For this review, take the finished solid that the model builds, in its own axes (mm). Face numbers are marked on the shaded views. A direction names the side the tool comes from. Give positions to 0.01 mm unless a question says otherwise; leave off trailing zeros. Loops run counter-clockwise (first coordinate to the right, second up) from the corner with the lowest first, then second, coordinate; pieces in that order, holes last. Notation, with made-up numbers: (46, -12.75) -> (88, -12.75) arc R21 ccw to (88, 3.25) -> close; hole circle Ø5 at (-25, 14). An arc over 180 degrees is marked (long way). Write each question's results on one line, items separated by ' | '. Start each with the question number.
```python
from build123d import *

# Parameters (mm, degrees)
SKETCH1_R           = 1.7
BOSS_EXTRUDE1_DEPTH = 34.5
CUT_EXTRUDE1_DEPTH  = 20.5
CUT_EXTRUDE2_START  = -7
CUT_EXTRUDE2_DEPTH  = 7


with BuildPart() as part:
    # Sketch1 → Boss-Extrude1 (new body)
    with BuildSketch(Plane.XY):
        with BuildLine():
            Line((-1.71, 8.48), (5.42, 8.48))
            ThreePointArc((5.42, 8.48), (8.934320702, 7.024320703), (10.39, 3.51))
            Line((10.39, 3.51), (10.39, -3.510005593))
            ThreePointArc((10.39, -3.510005593), (8.934320702, -7.024326295), (5.42, -8.480005593))
            Line((5.42, -8.480005593), (-1.71, -8.480005593))
            ThreePointArc((-1.71, -8.480005593), (-5.224320703, -7.024326295), (-6.68, -3.510005593))
            Line((-6.68, -3.510005593), (-6.68, 3.51))
            ThreePointArc((-6.68, 3.51), (-5.224320703, 7.024320703), (-1.71, 8.48))
        make_face()
        Circle(SKETCH1_R, mode=Mode.SUBTRACT)
        with BuildLine():
            Line((3.708402898, 2.999994407), (3.708402898, -2.999994407))
            ThreePointArc((3.708402898, -2.999994407), (3.854849507, -3.353547798), (4.208402898, -3.499994407))
            Line((4.208402898, -3.499994407), (4.808402898, -3.499994407))
            ThreePointArc((4.808402898, -3.499994407), (5.161956288, -3.353547798), (5.308402898, -2.999994407))
            Line((5.308402898, -2.999994407), (5.308402898, 2.999994407))
            ThreePointArc((5.308402898, 2.999994407), (5.161956288, 3.353547798), (4.808402898, 3.499994407))
            Line((4.808402898, 3.499994407), (4.208402898, 3.499994407))
            ThreePointArc((4.208402898, 3.499994407), (3.854849507, 3.353547798), (3.708402898, 2.999994407))
        make_face(mode=Mode.SUBTRACT)
    extrude(amount=BOSS_EXTRUDE1_DEPTH)

    # Sketch2 → Cut-Extrude1 (cut)
    with BuildSketch(Plane.XY.offset(34.5)):
        with BuildLine():
            Line((7.57000536, -3.509982547), (7.56999464, 3.510017453))
            ThreePointArc((7.56999464, 3.510017453), (6.94026805, 5.03028575), (5.419994641, 5.66))
            Line((5.419994641, 5.66), (-1.71000536, 5.66))
            ThreePointArc((-1.71000536, 5.66), (-3.230284939, 5.03027958), (-3.86000536, 3.51))
            Line((-3.86000536, 3.51), (-3.85999464, -3.51))
            ThreePointArc((-3.85999464, -3.51), (-3.230271899, -5.030278618), (-1.709991358, -5.659996717))
            Line((-1.709991358, -5.659996717), (5.420008642, -5.65998583))
            ThreePointArc((5.420008642, -5.65998583), (6.94028726, -5.030263088), (7.57000536, -3.509982547))
        make_face()
    extrude(amount=-CUT_EXTRUDE1_DEPTH, mode=Mode.SUBTRACT)

    # Sketch3 → Cut-Extrude2 (cut)
    with BuildSketch(Plane.XY.offset(14).offset(CUT_EXTRUDE2_START)):
        with BuildLine():
            Line((5.508402898, 3.499994407), (4.208402898, 3.499994407))
            ThreePointArc((4.208402898, 3.499994407), (3.854849507, 3.353547798), (3.708402898, 2.999994407))
            Line((3.708402898, 2.999994407), (3.708402898, -2.999994407))
            ThreePointArc((3.708402898, -2.999994407), (3.854849507, -3.353547798), (4.208402898, -3.499994407))
            Line((4.208402898, -3.499994407), (5.508402898, -3.499994407))
            ThreePointArc((5.508402898, -3.499994407), (5.861956288, -3.353547798), (6.008402898, -2.999994407))
            Line((6.008402898, -2.999994407), (6.008402898, 2.999994407))
            ThreePointArc((6.008402898, 2.999994407), (5.861956288, 3.353547798), (5.508402898, 3.499994407))
        make_face()
    extrude(amount=CUT_EXTRUDE2_DEPTH, mode=Mode.SUBTRACT)


solid = part.part
```
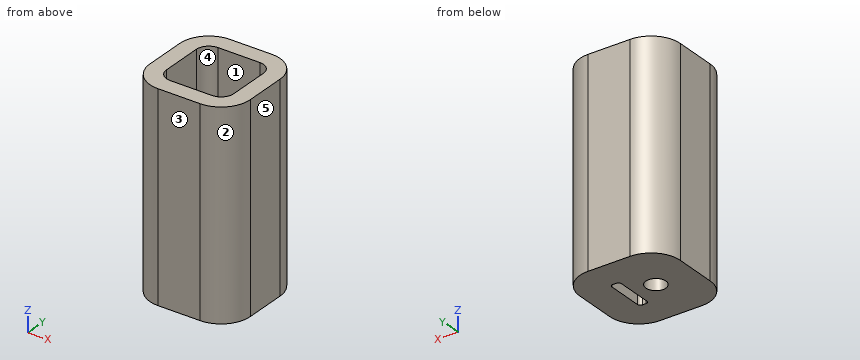
1. Draft analysis for pull direction X (two halves, no side actions). For the marked faces 3, 4 and 5, state which applies: released by +X, released by -X, zero draft, split by the parting line, or undercut.
2. We need section D-D (x = 0). Write out the cut boundary in (y, z), plus the area to 3 significant figures.
3. We need section B-B (z = 5). Write out the cut boundary in (x, y).
4. We need section C-C (y = 2.5). Write out the cut boundary in (x, z).
5. Machinability: for the marked faces 1 and 2, which of the approach directions +Z, -Z, +X, -X, +Y, -Y give a long, thin tool a straight path to every point of the face, cutting with its end or side? Answer none if there is none.
6. For pin 1 Ø2.5 at (x, y) = (0, 0) entering from -Z; pin 2 Ø9 at (x, y) = (1, 1) entering from +Z; pin 3 Ø3 at (x, y) = (5, -5) entering from +Z, all flat-tipped, find the tip position at first contact; note any pin that passes through.
7. Wall thickness on L1, parallel to X at y = 0, z = 5; L2, parallel to Y at x = 0, z = 3.5; L3, parallel to X at y = -2.5, z = 25: over which ranges is each line inside the solid? List them lowest first.
8. We need section A-A (y = 0). Write out the cut boundary in (x, z), plus the area to 3 significant figures.
Response:
1) face 3: zero draft | face 4: undercut | face 5: released by +X
2) outline: (-8.48, 0) -> (-1.7, 0) -> (-1.7, 14) -> (-5.66, 14) -> (-5.66, 34.5) -> (-8.48, 34.5) -> close; (1.7, 0) -> (8.48, 0) -> (8.48, 34.5) -> (5.66, 34.5) -> (5.66, 14) -> (1.7, 14) -> close | area: 305 mm2
3) outline: (-6.68, -3.51) arc R4.97 ccw to (-1.71, -8.48) -> (5.42, -8.48) arc R4.97 ccw to (10.39, -3.51) -> (10.39, 3.51) arc R4.97 ccw to (5.42, 8.48) -> (-1.71, 8.48) arc R4.97 ccw to (-6.68, 3.51) -> close; hole circle Ø3.4 at (0, 0); hole (3.71, -3) arc R0.5 ccw to (4.21, -3.5) -> (4.81, -3.5) arc R0.5 ccw to (5.31, -3) -> (5.31, 3) arc R0.5 ccw to (4.81, 3.5) -> (4.21, 3.5) arc R0.5 ccw to (3.71, 3) -> close
4) outline: (-6.68, 0) -> (3.71, 0) -> (3.71, 14) -> (-3.86, 14) -> (-3.86, 34.5) -> (-6.68, 34.5) -> close; (5.31, 0) -> (10.39, 0) -> (10.39, 34.5) -> (7.57, 34.5) -> (7.57, 14) -> (6.01, 14) -> (6.01, 7) -> (5.31, 7) -> close
5) face 1: +Z | face 2: +Z, -Z, +X, -Y
6) pin 1: passes through | pin 2: stops at z = 14 | pin 3: stops at z = 34.5
7) L1: x = -6.68 to -1.7, 1.7 to 3.71, 5.31 to 10.39 | L2: y = -8.48 to -1.7, 1.7 to 8.48 | L3: x = -6.68 to -3.86, 7.57 to 10.39
8) outline: (-6.68, 0) -> (-1.7, 0) -> (-1.7, 14) -> (-3.86, 14) -> (-3.86, 34.5) -> (-6.68, 34.5) -> close; (1.7, 0) -> (3.71, 0) -> (3.71, 14) -> (1.7, 14) -> close; (5.31, 0) -> (10.39, 0) -> (10.39, 34.5) -> (7.57, 34.5) -> (7.57, 14) -> (6.01, 14) -> (6.01, 7) -> (5.31, 7) -> close | area: 280 mm2
